Here's how the part is built. I have some questions about the finished solid (model axes, mm). Face numbers are marked on the shaded views. A direction names the side the tool comes from. Round coordinates to 2 decimals unless told otherwise and drop trailing zeros. Write each loop counter-clockwise with the first axis right and the second up, starting at its lowest first coordinate (ties: lowest second). Pieces come first, ordered by that corner, then holes. Notation, with made-up numbers: (-33, -24) - (-1, -24) arc R21 cw to (-1, -8) - close; hole circle Ø11 at (-17, -13.5). An arc over 180 degrees is marked (long way). One line per item, written item: value. Start each with the question number.
Item 1: Thinking about a two-plate mould opening in Y: for the marked faces 1, 2, 3 and 4, which applies, released by +Y, released by -Y, zero draft, split by the parting line, or undercut?
Item 2: For P1, Ø1.2, axis at y = 3, z = 0, coming from the +X side; P2, Ø2.5, axis at x = 3.5, z = -1.5, coming from the -Y side; P3, Ø4, axis at x = -4, z = -2, coming from the -Y side, each with a flat end and sliding along its axis, tell me the tip position at first contact or that it passes through.
Item 3: For the marked faces 5, 6 and 7, which set-ups out of +Z, -Z, +X, -X, +Y, -Y let a thin tool reach every point of the face, with its end or its side?
Item 4: Imagine slicing it at A-A, the plane y = 4. Please give me the cut outline in (x, z), then the cut area to 3 significant figures.
```python
from build123d import *

# Parameters (mm, degrees)
F0_W      = 16.9
F0_H      = 26
F1_DEPTH  = 6
F4_DEPTH  = 13
F5_R      = 0.5
F7_R      = 3.446906
F11_DEPTH = 12.001
F13_DEPTH = 8
F15_R     = 1.24365
F16_DEPTH = 5


with BuildPart() as f1:
    # F0 (on Right) → F1 (new body, symmetric)
    with BuildSketch(Plane.YZ):
        Rectangle(F0_W, F0_H)
    extrude(amount=F1_DEPTH, both=True)

    # F3 (on offset) → F4 (cut)
    with BuildSketch(Plane.XY.offset(13)):
        with BuildLine():
            Line((6, -3.679424), (6, -1.229189))
            ThreePointArc((6, -1.229189), (2.508033, -2.454307), (6, -3.679424))
        make_face()
    extrude(amount=-F4_DEPTH, mode=Mode.SUBTRACT)

    # F5 (on Top) → F8 section 0
    with BuildSketch(Plane.XY):
        with Locations((5.5, -2.421203)):
            Circle(F5_R)
    # F7 (on offset) → F8 section 1
    with BuildSketch(Plane.XY.offset(-13)):
        with Locations((0, -2.394957)):
            Circle(F7_R)
    loft(mode=Mode.SUBTRACT)

    # F10 (on offset) → F11 (cut, through all)
    with BuildSketch(Plane.YZ.offset(6)):
        with BuildLine():
            Line((8.45, -6.165668), (8.45, 5.995139))
            ThreePointArc((8.45, 5.995139), (7.398846, -0.085264), (8.45, -6.165668))
        make_face()
        with BuildLine():
            Line((-8.45, 5.754331), (-8.45, -6.406476))
            ThreePointArc((-8.45, -6.406476), (-7.398846, -0.326072), (-8.45, 5.754331))
        make_face()
    extrude(amount=-F11_DEPTH, mode=Mode.SUBTRACT)

    # F12 (on offset) → F13 (cut)
    with BuildSketch(Plane.YZ.offset(6)):
        with BuildLine():
            Line((1.735005, 13), (1.735005, -8.976745))
            ThreePointArc((1.735005, -8.976745), (3.66279, -11.704157), (5.590574, -8.976745))
            Line((5.590574, -8.976745), (5.590574, 13))
            Line((5.590574, 13), (1.735005, 13))
        make_face()
    extrude(amount=-F13_DEPTH, mode=Mode.SUBTRACT)

    # F15 (on offset) → F16 (cut)
    with BuildSketch(Plane.YZ.offset(2)):
        with Locations((3.523343, 0)):
            Circle(F15_R)
    extrude(amount=-F16_DEPTH, mode=Mode.SUBTRACT)


solid = f1.part
```
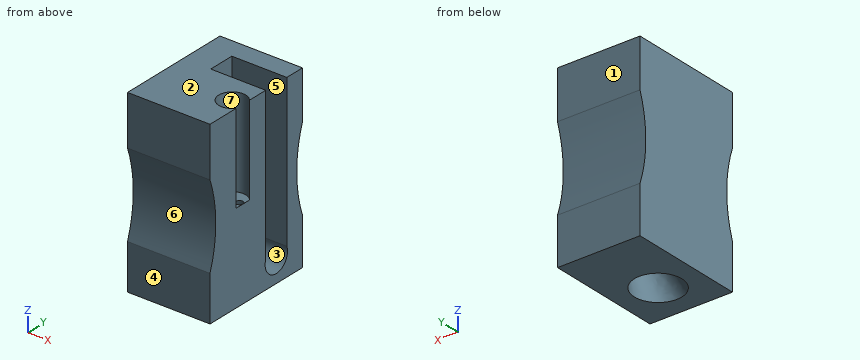
Values follow:
1. face 1: released by +Y
1. face 2: zero draft
1. face 3: undercut
1. face 4: released by -Y
2. P1: stops at x = -3
2. P2: stops at y = -7.56
2. P3: stops at y = -7.78
3. face 5: +Z, +X
3. face 6: +X, -X, -Y
3. face 7: +Z
4. outline: (-6, -13) - (6, -13) - (6, -11.68) - (-2, -11.68) - (-2, -1.15) - (-3, -1.15) - (-3, 1.15) - (-2, 1.15) - (-2, 13) - (-6, 13) - close
4. area: 112 mm^2
